Input: part model. Units: mm. Frame: model coordinates. Face numbers are marked on the shaded views. Coordinates: 2 decimals unless noted, no trailing zeros. Loops run counter-clockwise (first coordinate to the right, second up) from the corner with the lowest first, then second, coordinate; pieces in that order, holes last.
Item 1: Section A-A on y = 0. Return loops of the section in (x, z).
Item 2: Section B-B on z = 0. Return loops of the section in (x, y), and give its area (4 significant figures).
Item 3: Section D-D on x = -5.5. Give the number of separate pieces and of enclosed holes in the cut face, and give its area (3 significant figures).
Item 4: Contact query for flat-ended pins moving along their axis: P1, Ø1, axis at y = -2, z = 2, coming from the +X side; P2, Ø1, axis at x = -4, z = 2, coming from the -Y side; P3, Ø2.5, axis at y = -6, z = 0, coming from the +X side. Output: stop coordinate, or through.
Item 5: Ray query, line 1 along Z through (x, y) = (-1.75, -6); line 2 along Y through (x, z) = (-4, 0); line 3 along X through (y, z) = (-0.5, -2). Return the intervals inside material, ascending.
Item 6: Pull-direction query (Z, two-part tool) for the marked faces 1, 2, 3 and 4; classes: released by +Z, released by -Z, zero draft, split by the parting line, or undercut.
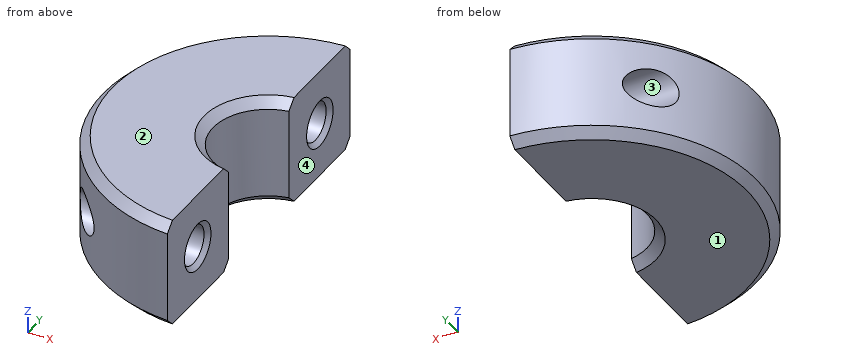
Autodesk Inventor part; units mm, degrees
ref_plane "2_1_XY" through (0, 0, 0) normal (1, 0, 0) x (0, 0, -1)
ref_plane "2_1_YZ" through (0, 0, 0) normal (0, 0, -1) x (0, 1, 0)
ref_plane "2_1_ZX" through (0, 0, 0) normal (0, 1, 0) x (1, 0, 0)
sketch "Sketch_1" plane through (0, 0, 0) normal (1, 0, 0) x (0, 1, 0)
  line L0 (0, -3) -> (0, 3)
  line L1 (8.5, 3) -> (3.5, 3)
  line L2 (3.5, 3) -> (3, 2.5)
  line L3 (3, 2.5) -> (3, -2.5)
  line L4 (3, -2.5) -> (3.5, -3)
  line L5 (3.5, -3) -> (8.5, -3)
  line L6 (8.5, -3) -> (9, -2.5)
  line L7 (9, -2.5) -> (9, 2.5)
  line L8 (9, 2.5) -> (8.5, 3)
revolve "Revolution1" add sketch "Sketch_1" angle 180 about axis through (0, 0, -3) along (0, 0, 1)
sketch "Sketch_2" plane through (0, 0, 0) normal (0, 0, 1) x (1, 0, 0)
  line L0 (-0.5, -10) -> (0.5, -10)
  line L1 (0.5, -10) -> (0.5, 10)
  line L2 (0.5, 10) -> (-0.5, 10)
  line L3 (-0.5, 10) -> (-0.5, -10)
extrude "Extrusion1" cut sketch "Sketch_2" along normal mid plane 6
sketch "Sketch3" plane through (-0.5, -8.4853, -3) normal (1, 0, 0) x (0, 0, -1)
  point P0 (-3, 2.4853)
hole "Hole1" at (-0.5, -6, 0) direction (-1, 0, 0) diameter 2.1129 depth 9 countersink diameter 2.6 countersink angle 90
sketch "Sketch4" plane through (-0.5, 3.4641, 3) normal (1, 0, 0) x (0, 0, -1)
  point P0 (3, 2.5359)
hole "Hole2" at (-0.5, 6, 0) direction (-1, 0, 0) diameter 2.1129 depth 9 countersink diameter 2.6 countersink angle 90
ref_plane "2_1_XY" through (0, 0, 0) normal (1, 0, 0) x (0, 0, -1)
ref_plane "2_1_YZ" through (0, 0, 0) normal (0, 0, -1) x (0, 1, 0)
ref_plane "2_1_ZX" through (0, 0, 0) normal (0, 1, 0) x (1, 0, 0)
properties part number "PSCSPJ6-6p"
Results found:
1. outline: (-9, -2.5) - (-8.5, -3) - (-3.5, -3) - (-3, -2.5) - (-3, 2.5) - (-3.5, 3) - (-8.5, 3) - (-9, 2.5) - close
2. outline: (-7.52, -4.94) - (-0.74, -4.94) - (-0.5, -4.7) - (-0.5, -2.96) arc R3 cw to (-0.5, 2.96) - (-0.5, 4.7) - (-0.74, 4.94) - (-7.52, 4.94) arc R9 ccw to start; (-5.59, -7.06) arc R9 ccw to (-0.5, -8.99) - (-0.5, -7.3) - (-0.74, -7.06) - close; (-5.59, 7.06) - (-0.74, 7.06) - (-0.5, 7.3) - (-0.5, 8.99) arc R9 ccw to start
2. area: 80.95 mm2
3. separate pieces: 1
3. enclosed holes: 2
3. area: 77.8 mm2
4. P1: stops at x = -1.66
4. P2: stops at y = -8.29
4. P3: stops at x = -0.55
5. line 1: z = -3 to -1.06, 1.06 to 3
5. line 2: y = -8.06 to -7.06, -4.94 to 4.94, 7.06 to 8.06
5. line 3: x = -8.99 to -2.96
6. face 1: released by -Z
6. face 2: released by +Z
6. face 3: undercut
6. face 4: zero draft
